from build123d import *

# Parameters (mm, degrees)
SKETCH_1_W          = 6.3
SKETCH_1_H          = 15
EXTRUDE_1_DEPTH     = 56
CUT_EXTRUDE_START   = -1.5
SKETCH_2_R          = 7.5
CUT_EXTRUDE_1_DEPTH = 53
CHAMFER_1_SIZE      = 0.5
CHAMFER_1_SIZE_2    = 0.37535302
CUT_EXTRUDE_5_DEPTH = 57


with BuildPart() as part:
    # 草图1 → 凸台-拉伸1 (new body)
    with BuildSketch(Plane.XY):
        with BuildLine():
            Line((16.32455532, -40), (20, -40))
            Line((20, -40), (20, 0))
            Line((20, 0), (16.32455532, 0))
            ThreePointArc((16.32455532, 0), (10, -10), (3.67544468, 0))
            Line((3.67544468, 0), (0, 0))
            Line((0, 0), (0, -40))
            Line((0, -40), (3.67544468, -40))
            ThreePointArc((3.67544468, -40), (10, -30), (16.32455532, -40))
        make_face()
        with Locations((10, -20)):
            Rectangle(SKETCH_1_W, SKETCH_1_H, mode=Mode.SUBTRACT)
    extrude(amount=EXTRUDE_1_DEPTH)

    # 草图2 → 切除-拉伸1 (cut)
    with BuildSketch(Plane.XY.offset(56).offset(CUT_EXTRUDE_START)):
        with Locations((10, -3)):
            Circle(SKETCH_2_R)
        with Locations((10, -37)):
            Circle(SKETCH_2_R)
    extrude(amount=-CUT_EXTRUDE_1_DEPTH, mode=Mode.SUBTRACT)

    # 倒角1
    # the kernel refuses this chamfer: 0.5, 0.37535302 mm, written as the material it takes off along each edge
    with BuildSketch(Plane(origin=(10, -37, 56), x_dir=(-0.8097393602715859, -0.5867897139750857, 0), z_dir=(0.5867897139750857, -0.8097393602715859, 0))) as chamfer_1_piece_1:
        Polygon((7, CHAMFER_1_SIZE), (7 + CHAMFER_1_SIZE, 0), (7, 0), align=None)
    revolve(axis=Axis((10, -37, 56), (0, 0, -1)), revolution_arc=251.859051953, mode=Mode.SUBTRACT)
    with BuildSketch(Plane(origin=(10, -37, 54.5), x_dir=(-0.8097393602715859, -0.5867897139750857, 0), z_dir=(0.5867897139750857, -0.8097393602715859, 0))) as chamfer_1_piece_2:
        Polygon((7 + CHAMFER_1_SIZE, 0), (7, -CHAMFER_1_SIZE), (7, 0), align=None)
    revolve(axis=Axis((10, -37, 54.5), (0, 0, -1)), revolution_arc=251.859051953, mode=Mode.SUBTRACT)
    with BuildSketch(Plane(origin=(10, -37, 1.5), x_dir=(-0.8097393602715859, -0.5867897139750857, 0), z_dir=(0.5867897139750857, -0.8097393602715859, 0))) as chamfer_1_piece_3:
        Polygon((7, CHAMFER_1_SIZE), (7 + CHAMFER_1_SIZE, 0), (7, 0), align=None)
    revolve(axis=Axis((10, -37, 1.5), (0, 0, -1)), revolution_arc=251.859051953, mode=Mode.SUBTRACT)
    with BuildSketch(Plane(origin=(10, -37, 0), x_dir=(-0.8097393602715859, -0.5867897139750857, 0), z_dir=(0.5867897139750857, -0.8097393602715859, 0))) as chamfer_1_piece_4:
        Polygon((7, -CHAMFER_1_SIZE), (7 + CHAMFER_1_SIZE, 0), (7, 0), align=None)
    revolve(axis=Axis((10, -37, 0), (0, 0, -1)), revolution_arc=251.859051953, mode=Mode.SUBTRACT)
    with BuildSketch(Plane(origin=(10, -3, 1.5), x_dir=(0.809739360271586, 0.5867897139750856, 0), z_dir=(-0.5867897139750856, 0.809739360271586, 0))) as chamfer_1_piece_5:
        Polygon((7, CHAMFER_1_SIZE), (7 + CHAMFER_1_SIZE, 0), (7, 0), align=None)
    revolve(axis=Axis((10, -3, 1.5), (0, 0, -1)), revolution_arc=251.859051953, mode=Mode.SUBTRACT)
    with BuildSketch(Plane(origin=(10, -3, 0), x_dir=(0.809739360271586, 0.5867897139750856, 0), z_dir=(-0.5867897139750856, 0.809739360271586, 0))) as chamfer_1_piece_6:
        Polygon((7, -CHAMFER_1_SIZE), (7 + CHAMFER_1_SIZE, 0), (7, 0), align=None)
    revolve(axis=Axis((10, -3, 0), (0, 0, -1)), revolution_arc=251.859051953, mode=Mode.SUBTRACT)
    with BuildSketch(Plane(origin=(10, -3, 56), x_dir=(0.809739360271586, 0.5867897139750855, 0), z_dir=(-0.5867897139750855, 0.809739360271586, 0))) as chamfer_1_piece_7:
        Polygon((7, CHAMFER_1_SIZE), (7 + CHAMFER_1_SIZE, 0), (7, 0), align=None)
    revolve(axis=Axis((10, -3, 56), (0, 0, -1)), revolution_arc=251.859051953, mode=Mode.SUBTRACT)
    with BuildSketch(Plane(origin=(10, -3, 54.5), x_dir=(0.809739360271586, 0.5867897139750855, 0), z_dir=(-0.5867897139750855, 0.809739360271586, 0))) as chamfer_1_piece_8:
        Polygon((7 + CHAMFER_1_SIZE, 0), (7, -CHAMFER_1_SIZE), (7, 0), align=None)
    revolve(axis=Axis((10, -3, 54.5), (0, 0, -1)), revolution_arc=251.859051953, mode=Mode.SUBTRACT)
    with BuildSketch(Plane(origin=(16.32455532, 0, 53.214158506), x_dir=(1, 0, 0), z_dir=(0, 0, 1)), Plane(origin=(3.67544468, -40, 53.214158506), x_dir=(-1, 0, 0), z_dir=(0, 0, 1))) as chamfer_1_piece_9:
        with BuildLine():
            Line((CHAMFER_1_SIZE, 0), (0.153157056, -0.346842944))
            ThreePointArc((0.153157056, -0.346842944), (0.080388037, -0.175694672), (0, 0))
            Line((0, 0), (CHAMFER_1_SIZE, 0))
        make_face()
    extrude(amount=4.071682988, mode=Mode.SUBTRACT)
    with BuildSketch(Plane(origin=(16.32455532, 0, -1.285841494), x_dir=(0.4039450974717048, -0.9147832301854768, 0), z_dir=(0, 0, 1)), Plane(origin=(3.67544468, -40, -1.285841494), x_dir=(-0.4039450974717028, 0.9147832301854776, 0), z_dir=(0, 0, 1))) as chamfer_1_piece_10:
        with BuildLine():
            Line((0.37915315, 0), (CHAMFER_1_SIZE * 0.403945097472, CHAMFER_1_SIZE * 0.914783230185))
            Line((CHAMFER_1_SIZE * 0.403945097472, CHAMFER_1_SIZE * 0.914783230185), (0, 0))
            ThreePointArc((0, 0), (0.193194893, 0.002566627), (0.37915315, 0))
        make_face()
    extrude(amount=4.071682988, mode=Mode.SUBTRACT)
    with BuildSketch(Plane(origin=(3.67544468, 0, -1.336191622), x_dir=(-1, 0, 0), z_dir=(0, 0, 1)), Plane(origin=(3.67544468, 0, 53.163808378), x_dir=(-1, 0, 0), z_dir=(0, 0, 1)), Plane(origin=(16.32455532, -40, -1.336191622), x_dir=(1, 0, 0), z_dir=(0, 0, 1)), Plane(origin=(16.32455532, -40, 53.163808378), x_dir=(1, 0, 0), z_dir=(0, 0, 1))) as chamfer_1_piece_11:
        with BuildLine():
            Line((CHAMFER_1_SIZE_2, 0), (0.205125138, 0.477447103))
            ThreePointArc((0.205125138, 0.477447103), (0.109888705, 0.243565694), (0, 0))
            Line((0, 0), (CHAMFER_1_SIZE_2, 0))
        make_face()
    extrude(amount=4.172383245, mode=Mode.SUBTRACT)

    # 草图3 → 切除-拉伸5 (cut)
    with BuildSketch(Plane.ZY):
        Polygon((25.8, -12.3), (30.2, -12.3), (33.2, -15.3), (33.2, -24.7), (30.2, -27.7), (25.8, -27.7), (22.8, -24.7), (22.8, -15.3), align=None)
    extrude(amount=-CUT_EXTRUDE_5_DEPTH, mode=Mode.SUBTRACT)


solid = part.part
Verification items for the finished model (mm, model axes). A direction names the side the tool comes from. Round coordinates to 2 decimals unless told otherwise and drop trailing zeros. Order: outer loops, then holes, each group sorted by start corner. A loop starts at its lowest first (then second) coordinate and runs counter-clockwise, first axis right, second up.
1. Section check A-A on y = -19. Record the cut outline in (x, z).
Final values:
outline: (0, 0) - (6.85, 0) - (6.85, 22.8) - (0, 22.8) - close; (0, 33.2) - (6.85, 33.2) - (6.85, 56) - (0, 56) - close; (13.15, 0) - (20, 0) - (20, 22.8) - (13.15, 22.8) - close; (13.15, 33.2) - (20, 33.2) - (20, 56) - (13.15, 56) - close
2. Section check D-D on y = -37. Record the cut outline in (x, z), then the cut area to 3 significant figures.
Final values:
outline: (0, 0) - (2.5, 0) - (3, 0.5) - (3, 1) - (2.5, 1.5) - (2.5, 54.5) - (3, 55) - (3, 55.5) - (2.5, 56) - (0, 56) - close; (17, 0.5) - (17.5, 0) - (20, 0) - (20, 56) - (17.5, 56) - (17, 55.5) - (17, 55) - (17.5, 54.5) - (17.5, 1.5) - (17, 1) - close
area: 282 mm2
3. Go/stop test with flat-tipped pins: P1, Ø7, axis at x = 9, z = 42.5, coming from the -Y side; P2, Ø7, axis at x = 9.5, z = 37, coming from the +Y side; P3, Ø1.3, axis at x = 5.5, z = 27.5, coming from the -Y side. Record where each tip stops, or that it passes through.
Final values:
P1: stops at y = -31
P2: stops at y = -9.34
P3: stops at y = -31.55
4. Section check C-C on z = 31. Record the cut outline in (x, y), then the cut area to 3 significant figures.
Final values:
outline: (0, -40) - (3.13, -40) arc R7.5 cw (long way) to (16.87, -40) - (20, -40) - (20, -26.9) - (13.15, -26.9) - (13.15, -27.5) - (6.85, -27.5) - (6.85, -26.9) - (0, -26.9) - close; (0, -13.1) - (6.85, -13.1) - (6.85, -12.5) - (13.15, -12.5) - (13.15, -13.1) - (20, -13.1) - (20, 0) - (16.87, 0) arc R7.5 cw (long way) to (3.13, 0) - (0, 0) - close
area: 252 mm2
5. Section check B-B on x = 10. Record the cut outline in (y, z).
Final values:
outline: (-30, 0.5) - (-29.5, 0) - (-27.5, 0) - (-27.5, 25.6) - (-27.7, 25.8) - (-27.7, 30.2) - (-27.5, 30.4) - (-27.5, 56) - (-29.5, 56) - (-30, 55.5) - (-30, 55) - (-29.5, 54.5) - (-29.5, 1.5) - (-30, 1) - close; (-12.5, 0) - (-10.5, 0) - (-10, 0.5) - (-10, 1) - (-10.5, 1.5) - (-10.5, 54.5) - (-10, 55) - (-10, 55.5) - (-10.5, 56) - (-12.5, 56) - (-12.5, 30.4) - (-12.3, 30.2) - (-12.3, 25.8) - (-12.5, 25.6) - close
6. Thickness scan on L1, parallel to X at y = -37, z = 55; L2, parallel to X at y = -37, z = 43.5; L3, parallel to Z at x = 3.25, y = -19.5. Record the ranges inside material, lowest first.
Final values:
L1: x = 0 to 3, 17 to 20
L2: x = 0 to 2.5, 17.5 to 20
L3: z = 0 to 22.8, 33.2 to 56
7. Release check for a two-part mould opening along Z. For faces 4 (the flat face through (10, -12.3, 28)), 5 (the conical face through (9.83, -29.86, 55.64)), 6 (the flat face through (18, -40, 28)) record: +Z half, -Z half, draft (parallel to the pull), parting line (faces both ways), or undercut.
Final values:
face 4: undercut
face 5: +Z half
face 6: draft
8. Access from +Z, -Z, +X, -X, +Y, -Y to the whole of each face (thin tool, end or side, straight path). Record for faces 1 (the flat face through (13.15, -20, 13)), 2 (the flat face through (3, -20, 22.8)), 3 (the cylindrical face through (10.208, -29.503, 28.371)).
Final values:
face 1: +Z, -Z
face 2: +X, -X
face 3: none
